The figure shows three views and two pictorial views of one solid part (mm, origin at its lowest corner). Answer the questions. Coordinates: 2 decimals unless noted, no trailing zeros. Order: outer loops, then holes, each group sorted by start corner. A loop starts at its lowest first (then second) coordinate and runs counter-clockwise, first axis right, second up. Notation, with made-up numbers: (66.25, -3.75) -> (103.25, -3.75) arc R27 cw to (103.25, 24.25) -> close; hole circle Ø2 at (16.25, -23). An arc over 180 degrees is marked (long way). Return JSON: item names as keys, results as strings.
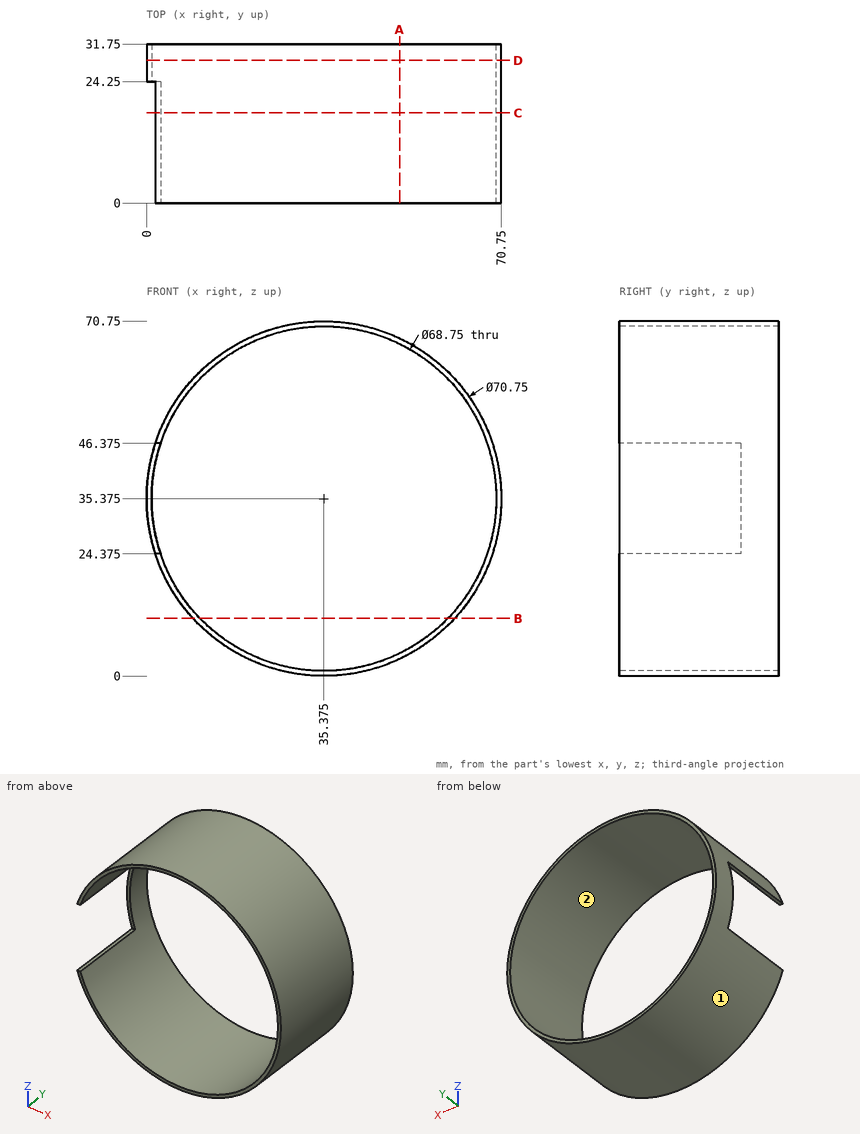
1. The part is cut by section D-D on y = 28.5. Give the vertices of the cut face in (x, z) (3 decimals).
Answer block:
{"outline": "circle Ø70.75 at (35.375, 35.375); hole circle Ø68.75 at (35.375, 35.375)"}
2. Consider line 1 (X direction, y = 27, z = 28); line 2 (Z direction, x = 58.5, y = 12.5); line 3 (X direction, y = 13, z = 67). Determine where each line is inside the solid, lowest interval first. Write a range as from..to.
Answer block:
{"line 1": "x = 0.78..1.8, 68.95..69.97", "line 2": "z = 8.61..9.94, 60.81..62.14", "line 3": "x = 19.52..21.9, 48.85..51.23"}
3. The part is cut by section C-C on y = 18. Give the vertices of the cut face in (x, z) (3 decimals).
Answer block:
{"outline": "(1.754, 24.375) arc R35.375 ccw (long way) to (1.754, 46.375) -> (2.808, 46.375) arc R34.375 cw (long way) to (2.808, 24.375) -> close"}
4. Each of these flat-tipped pins is pushed along its axis until it touches: pin 1 Ø10 at (y, z) = (22.5, 24.5) entering from -X; pin 2 Ø5 at (y, z) = (21, 24) entering from -X; pin 3 Ø5 at (x, y) = (53, 27.5) entering from +Z. Where does it stop, or does it pass through?
Answer block:
{"pin 1": "stops at x = 0.55", "pin 2": "stops at x = 1.75", "pin 3": "stops at z = 67.35"}
5. The part is cut by section B-B on z = 11.5. Give the vertices of the cut face in (x, y), and give its area (3 significant figures).
Answer block:
{"outline": "(9.27, 0) -> (10.64, 0) -> (10.64, 31.75) -> (9.27, 31.75) -> close; (60.11, 0) -> (61.48, 0) -> (61.48, 31.75) -> (60.11, 31.75) -> close", "area": "87.1 mm2"}
6. Determine the mould class of the marked faces 1 and 2 for opening direction X: pulls with the +X half, pulls with the -X half, needs draft (parallel to the pull), parting line crosses it, or undercut.
Answer block:
{"face 1": "parting line crosses it", "face 2": "undercut"}
7. The part is cut by section A-A on x = 50.5. Give the vertices of the cut face in (y, z).
Answer block:
{"outline": "(0, 3.4) -> (31.75, 3.4) -> (31.75, 4.51) -> (0, 4.51) -> close; (0, 66.24) -> (31.75, 66.24) -> (31.75, 67.35) -> (0, 67.35) -> close"}
